Can you work these out from the model? Positions are in its coordinate system, mm. A direction names the side the tool comes from. Round coordinates to 2 decimals unless told otherwise and drop trailing zeros. Write each loop counter-clockwise with the first axis right and the second up, starting at its lowest first coordinate (ties: lowest second). Pieces come first, ordered by that corner, then holes.
Q1. I'm going to push flat-ended pins straight in: pin 1 Ø1 at (x, z) = (-24.5, 2.5) entering from +Y; pin 2 Ø3 at (x, y) = (7, -20.5) entering from -Z. Where does each tip first touch, or does it pass through?
Q2. If we section it at D-D (x = -1): Please give me the cut outline in (y, z), plus the area to 3 significant figures.
Q3. For faces 5 (the flat face through (0, 0, 10)), 6 (the cylindrical face through (-33.5, 31.3, 4.9)), which set-ups out of +Z, -Z, +X, -X, +Y, -Y let a thin tool reach every point of the face, with its end or its side?
Q4. Please list where these lines run through material, in increasing order: line 1 along Z through (x, y) = (-31, -27); line 2 along X through (y, z) = (-25.9, 5); line 3 along Y through (x, z) = (-14, 4.25).
Q5. If we section it at B-B (x = -31): Please give me the cut outline in (y, z).
Q6. If we section it at A-A (z = 5): Please give me the cut outline in (x, y), plus the area to 4 significant figures.
Q7. If we section it at C-C (z = 1): Please give me the cut outline in (x, y).
Q8. We'd pull the mould along X, two halves only. Please class faces 1 (the flat face through (-31, -25, 5)), 2 (the cylindrical face through (-33.5, -26.3, 5.1)), 3 (the flat face through (0, 0, 0)), 4 (the flat face through (-35, 0, 5)): +X half, -X half, draft (parallel to the pull), parting line (faces both ways), or undercut.
from build123d import *

# Parameters (mm, degrees)
SKETCH1_W           = 70
SKETCH1_H           = 55
BOSS_EXTRUDE1_DEPTH = 10
SKETCH2_R           = 2.5
BOSS_EXTRUDE2_DEPTH = 35
SKETCH3_R           = 2.5
CUT_EXTRUDE1_DEPTH  = 10


with BuildPart() as part:
    # Sketch1 → Boss-Extrude1 (new body)
    with BuildSketch(Plane.XY):
        Rectangle(SKETCH1_W, SKETCH1_H)
    extrude(amount=BOSS_EXTRUDE1_DEPTH)

    # Sketch2 → Boss-Extrude2 (add, symmetric)
    with BuildSketch(Plane(origin=(0, 0, 0), x_dir=(1, 0, 0), z_dir=(0, 1, 0))):
        with Locations((-31, -5)):
            Circle(SKETCH2_R)
    extrude(amount=BOSS_EXTRUDE2_DEPTH, both=True)

    # Sketch3 → Cut-Extrude1 (cut)
    with BuildSketch(Plane.XZ.offset(35)):
        with Locations((-31, 5)):
            Circle(SKETCH3_R)
    extrude(amount=-CUT_EXTRUDE1_DEPTH, mode=Mode.SUBTRACT)


solid = part.part
A:
1. pin 1: stops at y = 27.5
1. pin 2: stops at z = 0
2. outline: (-27.5, 0) - (27.5, 0) - (27.5, 10) - (-27.5, 10) - close
2. area: 550 mm2
3. face 5: +Z, +X, -X, +Y, -Y
3. face 6: +Y
4. line 1: z = 0 to 2.5, 7.5 to 10
4. line 2: x = -35 to -33.5, -28.5 to 35
4. line 3: y = -27.5 to 27.5
5. outline: (-27.5, 0) - (27.5, 0) - (27.5, 2.5) - (35, 2.5) - (35, 7.5) - (27.5, 7.5) - (27.5, 10) - (-27.5, 10) - (-27.5, 7.5) - (-25, 7.5) - (-25, 2.5) - (-27.5, 2.5) - close
6. outline: (-35, -27.5) - (-33.5, -27.5) - (-33.5, -25) - (-28.5, -25) - (-28.5, -27.5) - (35, -27.5) - (35, 27.5) - (-28.5, 27.5) - (-28.5, 35) - (-33.5, 35) - (-33.5, 27.5) - (-35, 27.5) - close
6. area: 3,875 mm2
7. outline: (-35, -27.5) - (35, -27.5) - (35, 27.5) - (-35, 27.5) - close
8. face 1: undercut
8. face 2: undercut
8. face 3: draft
8. face 4: -X half
